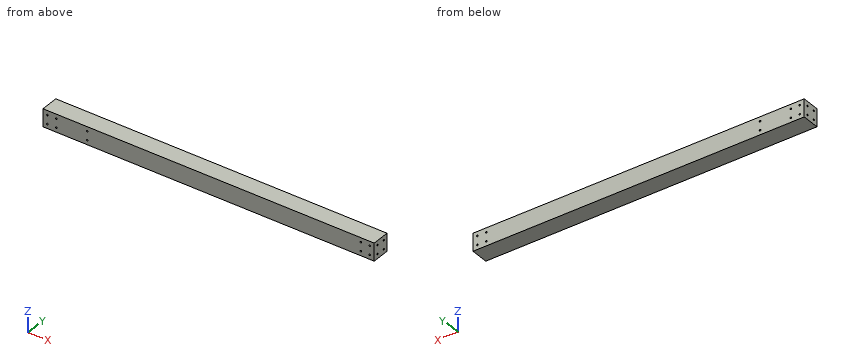
```python
from build123d import *

# Parameters (mm, degrees)
F0_W     = 60
F0_H     = 60
F1_DEPTH = 1124
F2_D     = 5.5
F4_D     = 5.5
F5_D     = 5.5


with BuildPart() as f1:
    # F0 (on Right) → F1 (new body)
    with BuildSketch(Plane.YZ):
        with Locations((-30, 30)):
            Rectangle(F0_W, F0_H)
    extrude(amount=F1_DEPTH)

    # F2 (through all)
    with Locations(Plane(origin=(0, 0, 0), x_dir=(0, 1, 0), z_dir=(-1, 0, 0))):
        with Locations((-45, -45), (-45, -15), (-15, -15), (-15, -45)):
            Hole(F2_D / 2)

    # F4 (through all)
    with Locations(Plane.XZ.offset(60)):
        with Locations((150, 45), (150, 15)):
            Hole(F4_D / 2)

    # F5 (through all)
    with Locations(Plane.XZ.offset(60)):
        with Locations((45, 45), (15, 45), (15, 15), (45, 15), (1109, 45), (1079, 15), (1109, 15), (1079, 45)):
            Hole(F5_D / 2)


solid = f1.part
```
Geometry: final body of the model. Coordinates: model frame, mm. Round coordinates to 2 decimals unless told otherwise and drop trailing zeros. Write each loop counter-clockwise with the first axis right and the second up, starting at its lowest first coordinate (ties: lowest second). Pieces come first, ordered by that corner, then holes. Notation, with made-up numbers: M 33,36.25 L 69,36.25 A23 ccw 69,67.25 Z; hole C -38,67 d1. An arc over 180 degrees is marked long. Answer in a Markdown table with one row per item. Add a question column.
(1) Cut plane A-A, the plane x = 494.5. Return the cut outline in (y, z), then the cut area to 3 significant figures.
(2) Contact query for a flat-ended pin moving along its axis: pin 1 (5 mm diameter, centred on x = 15, z = 15, fed in from +Y). Output: stop coordinate, or through.
(3) Ray query, L1, parallel to Y at x = 10.75, z = 15; L2, parallel to Z at x = 1087, y = -15; L3, parallel to X at y = -22, z = 15. Return the intervals inside material, ascending.
Established:
| question | item | result |
|---|---|---|
| 1 | outline | M -60,0 L 0,0 L 0,60 L -60,60 Z; hole C -45,15 d5.5; hole C -45,45 d5.5; hole C -15,15 d5.5; hole C -15,45 d5.5 |
| 1 | area | 3,500 mm² |
| 2 | pin 1 | through |
| 3 | L1 | -60 to -47.75, -42.25 to -17.75, -12.25 to 0 |
| 3 | L2 | 0 to 12.25, 17.75 to 42.25, 47.75 to 60 |
| 3 | L3 | 0 to 12.25, 17.75 to 42.25, 47.75 to 147.25, 152.75 to 1076.25, 1081.75 to 1106.25, 1111.75 to 1124 |
